from build123d import *

# Parameters (mm, degrees)
CYLINDER_R        = 1.6
CYLINDER_DEPTH    = 10
BOX001_W          = 7.5
BOX001_H          = 7.5
BOX001_DEPTH      = 3
FILLET002_R       = 3.5
FILLET003_R       = 3.5
CYLINDER005_R     = 1.5
CYLINDER005_DEPTH = 10
CYLINDER004_R     = 1.5
CYLINDER004_DEPTH = 10
CYLINDER003_R     = 1.5
CYLINDER003_DEPTH = 10
CYLINDER002_R     = 1.5
CYLINDER002_DEPTH = 10
BOX_W             = 15
BOX_H             = 42
BOX_DEPTH         = 3
CHAMFER005_SIZE   = 11.8
CHAMFER006_SIZE   = 11.8
PAD_DEPTH         = 5
CHAMFER_SIZE      = 1
CHAMFER001_SIZE   = 1
CHAMFER002_SIZE   = 1
CHAMFER003_SIZE   = 2
CHAMFER004_SIZE   = 2
CYLINDER001_R     = 1.6
CYLINDER001_DEPTH = 10
BOX002_W          = 7.5
BOX002_H          = 7.5
BOX002_DEPTH      = 3
FILLET_R          = 3.5
FILLET001_R       = 3.5


with BuildPart() as cylinder:
    # Cylinder → Cylinder (new body)
    with BuildSketch(Plane(origin=(-4, 4, 0), x_dir=(1, 0, 0), z_dir=(0, 0, 1))):
        Circle(CYLINDER_R)
    extrude(amount=CYLINDER_DEPTH)


with BuildPart() as cut001:
    # Box001 → Box001 (new body)
    with BuildSketch(Plane(origin=(-7.5, 0, 0), x_dir=(1, 0, 0), z_dir=(0, 0, 1))):
        with Locations((3.75, 3.75)):
            Rectangle(BOX001_W, BOX001_H)
    extrude(amount=BOX001_DEPTH)

    # Fillet002
    fillet002_edges = [cut001.edges().sort_by_distance(p)[0] for p in [
        (-7.5, 7.5, 1.5),
    ]]
    fillet(fillet002_edges, radius=FILLET002_R)

    # Fillet003
    fillet003_edges = [cut001.edges().sort_by_distance(p)[0] for p in [
        (-7.5, 0, 1.5),
    ]]
    fillet(fillet003_edges, radius=FILLET003_R)

    # Cut001: cut Cylinder
    add(cylinder.part, mode=Mode.SUBTRACT)


with BuildPart() as cylinder005:
    # Cylinder005 → Cylinder005 (new body)
    with BuildSketch(Plane(origin=(5, 18.5, 0), x_dir=(1, 0, 0), z_dir=(0, 0, 1))):
        Circle(CYLINDER005_R)
    extrude(amount=CYLINDER005_DEPTH)


with BuildPart() as cylinder004:
    # Cylinder004 → Cylinder004 (new body)
    with BuildSketch(Plane(origin=(5, 23.5, 0), x_dir=(1, 0, 0), z_dir=(0, 0, 1))):
        Circle(CYLINDER004_R)
    extrude(amount=CYLINDER004_DEPTH)


with BuildPart() as cylinder003:
    # Cylinder003 → Cylinder003 (new body)
    with BuildSketch(Plane(origin=(5, 28.5, 0), x_dir=(1, 0, 0), z_dir=(0, 0, 1))):
        Circle(CYLINDER003_R)
    extrude(amount=CYLINDER003_DEPTH)


with BuildPart() as cylinder002:
    # Cylinder002 → Cylinder002 (new body)
    with BuildSketch(Plane(origin=(5, 13.5, 0), x_dir=(1, 0, 0), z_dir=(0, 0, 1))):
        Circle(CYLINDER002_R)
    extrude(amount=CYLINDER002_DEPTH)


with BuildPart() as cut005:
    # Box → Box (new body)
    with BuildSketch(Plane.XY):
        with Locations((7.5, 21)):
            Rectangle(BOX_W, BOX_H)
    extrude(amount=BOX_DEPTH)

    # Chamfer005
    chamfer005_edges = [cut005.edges().sort_by_distance(p)[0] for p in [
        (15, 42, 1.5),
    ]]
    chamfer(chamfer005_edges, length=CHAMFER005_SIZE)

    # Chamfer006
    chamfer006_edges = [cut005.edges().sort_by_distance(p)[0] for p in [
        (15, 0, 1.5),
    ]]
    chamfer(chamfer006_edges, length=CHAMFER006_SIZE)

    # Cut002: cut Cylinder002
    add(cylinder002.part, mode=Mode.SUBTRACT)

    # Cut003: cut Cylinder003
    add(cylinder003.part, mode=Mode.SUBTRACT)

    # Cut004: cut Cylinder004
    add(cylinder004.part, mode=Mode.SUBTRACT)

    # Cut005: cut Cylinder005
    add(cylinder005.part, mode=Mode.SUBTRACT)


with BuildPart() as chamfer004:
    # Sketch → Pad (new body)
    with BuildSketch(Plane(origin=(-25, 21, 0), x_dir=(1, 0, 0), z_dir=(0, 0, 1))):
        with BuildLine():
            ThreePointArc((66.744349, -15.409147), (67.183792, -13.363687), (67.560564, -11.305761))
            Line((67.560564, -11.305761), (69.039992, -11.553332))
            ThreePointArc((69.039992, -11.553332), (70, 0), (69.039992, 11.553332))
            Line((67.560564, 11.305761), (69.039992, 11.553332))
            ThreePointArc((67.560564, 11.305761), (67.183792, 13.363687), (66.744349, 15.409147))
            Line((40, 9.234728), (66.744349, 15.409147))
            Line((40, 9.234728), (40, 6.693704))
            Line((40, 6.693704), (62.135993, 10.397999))
            ThreePointArc((62.135993, -10.397999), (63, 0), (62.135993, 10.397999))
            Line((40, -6.693704), (62.135993, -10.397999))
            Line((40, -6.693704), (40, -9.234728))
            Line((40, -9.234728), (66.744349, -15.409147))
        make_face()
    extrude(amount=PAD_DEPTH)

    # Chamfer
    chamfer_edges = [chamfer004.edges().sort_by_distance(p)[0] for p in [
        (42.183792, 34.363687, 5),
    ]]
    chamfer(chamfer_edges, length=CHAMFER_SIZE)

    # Chamfer001
    chamfer001_edges = [chamfer004.edges().sort_by_distance(p)[0] for p in [
        (45, 21, 5),
    ]]
    chamfer(chamfer001_edges, length=CHAMFER001_SIZE)

    # Chamfer002
    chamfer002_edges = [chamfer004.edges().sort_by_distance(p)[0] for p in [
        (42.183792, 7.636313, 5),
    ]]
    chamfer(chamfer002_edges, length=CHAMFER002_SIZE)

    # Chamfer003
    chamfer003_edges = [chamfer004.edges().sort_by_distance(p)[0] for p in [
        (15, 28.964216, 5),
    ]]
    chamfer(chamfer003_edges, length=CHAMFER003_SIZE)

    # Chamfer004
    chamfer004_edges = [chamfer004.edges().sort_by_distance(p)[0] for p in [
        (15, 13.035784, 5),
    ]]
    chamfer(chamfer004_edges, length=CHAMFER004_SIZE)


with BuildPart() as cylinder001:
    # Cylinder001 → Cylinder001 (new body)
    with BuildSketch(Plane(origin=(-4, 38, 0), x_dir=(1, 0, 0), z_dir=(0, 0, 1))):
        Circle(CYLINDER001_R)
    extrude(amount=CYLINDER001_DEPTH)


with BuildPart() as fusion:
    # Box002 → Box002 (new body)
    with BuildSketch(Plane(origin=(-7.5, 34.5, 0), x_dir=(1, 0, 0), z_dir=(0, 0, 1))):
        with Locations((3.75, 3.75)):
            Rectangle(BOX002_W, BOX002_H)
    extrude(amount=BOX002_DEPTH)

    # Fillet
    fillet_edges = [fusion.edges().sort_by_distance(p)[0] for p in [
        (-7.5, 34.5, 1.5),
    ]]
    fillet(fillet_edges, radius=FILLET_R)

    # Fillet001
    fillet001_edges = [fusion.edges().sort_by_distance(p)[0] for p in [
        (-7.5, 42, 1.5),
    ]]
    fillet(fillet001_edges, radius=FILLET001_R)

    # Cut: cut Cylinder001
    add(cylinder001.part, mode=Mode.SUBTRACT)

    # Fusion: union Cut001, Cut005, Chamfer004
    add(cut001.part)
    add(cut005.part)
    add(chamfer004.part)


solid = fusion.part
Verification items for the finished model (mm, model axes). A direction names the side the tool comes from. Coordinates: 2 decimals unless noted, no trailing zeros. Loops run counter-clockwise (first coordinate to the right, second up) from the corner with the lowest first, then second, coordinate; pieces in that order, holes last. Notation, with made-up numbers: (25.5, 74.5) -> (78.5, 74.5) arc R22 cw to (78.5, 97.5) -> close; hole circle Ø9 at (23, 11). An arc over 180 degrees is marked (long way). Answer as a JSON object with one key per item and string values. Group by question number.
Item 1: Depth check by flat-ended pin: pin 1 (5 mm diameter, centred on x = -4, y = 38, fed in from +Z); pin 2 (3 mm diameter, centred on x = 29.5, z = 1, fed in from -Y); pin 3 (0.9 mm diameter, centred on y = 24.5, z = 2, fed in from +X). Enter the tip coordinate at first touch or a pass-through.
Item 2: Sectioned sample at A-A on x = 33. Record the boundary of the cut face in (y, z), plus the area to 3 significant figures.
Item 3: Sectioned sample at C-C on x = 9. Record the boundary of the cut face in (y, z).
Item 4: Tool access check on faces 4 (the flat face through (9, 36.2, 1.5)), 5 (the flat face through (28.185, 8.721, 2.465)), 6 (the flat face through (15, 21, 1)), 7 (the flat face through (-2, 7.5, 1)). Record the directions out of +Z, -Z, +X, -X, +Y, -Y that give a thin tool (end or side, any length) a straight path to the whole face; none if there is none.
Item 5: Sectioned sample at B-B on y = 23.5. State how many separate pieces and enclosed holes the cut face has, plus the area to 3 significant figures.
Item 6: Mould release check, pull along X, two halves, no side actions. Record for faces 1 (the flat face through (0, 0, 1)), 2 (the flat face through (16, 29, 4)), 3 (the flat face through (43.338, 32.436, 2.465)): +X half, -X half, draft (parallel to the pull), parting line (faces both ways), or undercut.
Item 7: Sectioned sample at D-D on x = 26.5. Record the boundary of the cut face in (y, z), plus the area to 3 significant figures.
Item 8: Scan lines: probe 1 along Y at (x, z) = (-4, 1.9); probe 2 along X at (y, z) = (18, 1.4); probe 3 along Y at (x, z) = (5, 1.9). Record each from-to range of solid material in increasing order.
Evaluation:
{
 "1": {"pin 1": "stops at z = 3", "pin 2": "stops at y = 8.07", "pin 3": "stops at x = 44.93"},
 "2": {"outline": "(7.61, 0) -> (11.29, 0) -> (11.29, 5) -> (7.61, 5) -> close; (30.71, 0) -> (34.39, 0) -> (34.39, 5) -> (30.71, 5) -> close", "area": "36.8 mm²"},
 "3": {"outline": "(5.8, 0) -> (36.2, 0) -> (36.2, 3) -> (5.8, 3) -> close"},
 "4": {"face 4": "+Z, -Z, +Y", "face 5": "+Z, -Z, -Y", "face 6": "+Z, -Z", "face 7": "+Z, -Z, -X"},
 "5": {"separate pieces": "3", "enclosed holes": "0", "area": "70.5 mm²"},
 "6": {"face 1": "draft", "face 2": "-X half", "face 3": "undercut"},
 "7": {"outline": "(9.11, 0) -> (12.38, 0) -> (12.38, 5) -> (9.11, 5) -> close; (29.62, 0) -> (32.89, 0) -> (32.89, 5) -> (29.62, 5) -> close", "area": "32.7 mm²"},
 "8": {"probe 1": "y = 0 to 2.4, 5.6 to 7.5, 34.5 to 36.4, 39.6 to 42", "probe 2": "x = 0 to 3.59, 6.41 to 15, 37.93 to 44.94", "probe 3": "y = 1.8 to 12, 15 to 17, 20 to 22, 25 to 27, 30 to 40.2"}
}
